Work out the finished part from the listing and answer in its coordinate system (mm). A direction names the side the tool comes from. Coordinates: 2 decimals unless noted, no trailing zeros. Order: outer loops, then holes, each group sorted by start corner. A loop starts at its lowest first (then second) coordinate and runs counter-clockwise, first axis right, second up. Notation, with made-up numbers: M 81,-2 L 119,-2 A17 ccw 119,19 Z; hole C 48,-38.5 d11. An arc over 180 degrees is marked long. Use a Markdown table: item, result.
from build123d import *

# Parameters (mm, degrees)
SKETCH_1_W          = 40.6
SKETCH_1_H          = 20
EXTRUDE_1_DEPTH     = 2
SKETCH_2_W          = 2
SKETCH_2_H          = 20
EXTRUDE_2_DEPTH     = 22
SKETCH_3_R          = 2.5
CUT_EXTRUDE_1_DEPTH = 49.211616857


with BuildPart() as part:
    # 草图1 → 凸台-拉伸1 (new body)
    with BuildSketch(Plane.XY):
        Rectangle(SKETCH_1_W, SKETCH_1_H)
    extrude(amount=EXTRUDE_1_DEPTH)

    # 草图2 → 凸台-拉伸2 (add)
    with BuildSketch(Plane.XY.offset(2)):
        with Locations((-19.3, 0)):
            Rectangle(SKETCH_2_W, SKETCH_2_H)
        with Locations((19.3, 0)):
            Rectangle(SKETCH_2_W, SKETCH_2_H)
    extrude(amount=EXTRUDE_2_DEPTH)

    # 草图3 → 切除-拉伸1 (cut, through all)
    with BuildSketch(Plane.ZY.offset(20.3)):
        with Locations(Location((14, 0, 0), (0, 0, 270))):
            Circle(SKETCH_3_R)
    extrude(amount=-CUT_EXTRUDE_1_DEPTH, mode=Mode.SUBTRACT)


solid = part.part
(1) A cutting plane is placed at A-A (z = 12.5). Determine the outline of the cut face in (x, y), then the cut area to 3 significant figures.
Conclusion:
| item | result |
|---|---|
| outline | M -20.3,-10 L -18.3,-10 L -18.3,-2 L -20.3,-2 Z; M -20.3,2 L -18.3,2 L -18.3,10 L -20.3,10 Z; M 18.3,-10 L 20.3,-10 L 20.3,-2 L 18.3,-2 Z; M 18.3,2 L 20.3,2 L 20.3,10 L 18.3,10 Z |
| area | 64.0 mm2 |
(2) Determine the mould class of faces 1 (the flat face through (18.3, -2.4, 12.8)), 2 (the cylindrical face through (-19.31, 0.54, 11.56)), 3 (the flat face through (0, 0, 2)) for opening direction Z: pulls with the +Z half, pulls with the -Z half, needs draft (parallel to the pull), parting line crosses it, or undercut.
Conclusion:
| item | result |
|---|---|
| face 1 | needs draft |
| face 2 | undercut |
| face 3 | pulls with the +Z half |
(3) Which of the six approach directions +Z, -Z, +X, -X, +Y, -Y give full straight-line access (tool end or side, diameter ignored) to faces 4 (the flat face through (19, 0, 24)), 5 (the flat face through (-18.3, -2.4, 12.8))?
Conclusion:
| item | result |
|---|---|
| face 4 | +Z, +X, -X, +Y, -Y |
| face 5 | +Z, +Y, -Y |
(4) A cutting plane is placed at B-B (y = 0). Determine the outline of the cut face in (x, z), then the cut area to 3 significant figures.
Conclusion:
| item | result |
|---|---|
| outline | M -20.3,0 L 20.3,0 L 20.3,11.5 L 18.3,11.5 L 18.3,2 L -18.3,2 L -18.3,11.5 L -20.3,11.5 Z; M -20.3,16.5 L -18.3,16.5 L -18.3,24 L -20.3,24 Z; M 18.3,16.5 L 20.3,16.5 L 20.3,24 L 18.3,24 Z |
| area | 149 mm2 |
(5) Straight lines are drawn through the part: L1, parallel to Z at x = -19.45, y = 0; L2, parallel to X at y = 6, z = 6.5; L3, parallel to Z at x = -14.5, y = -8.5. For each, find the intervals that lie inside material, in ascending order.
Conclusion:
| item | result |
|---|---|
| L1 | 0 to 11.5, 16.5 to 24 |
| L2 | -20.3 to -18.3, 18.3 to 20.3 |
| L3 | 0 to 2 |
(6) Given P1, Ø1.5, axis at x = 1.5, y = 2.5, coming from the +Z side; P2, Ø8, axis at y = 0, z = 14, coming from the +X side, each flat-ended and moving along its own axis, determine where each tip first touches the part or whether it passes through.
Conclusion:
| item | result |
|---|---|
| P1 | z = 2 |
| P2 | x = 20.3 |
(7) A cutting plane is placed at C-C (z = 18). Determine the outline of the cut face in (x, y), then the cut area to 3 significant figures.
Conclusion:
| item | result |
|---|---|
| outline | M -20.3,-10 L -18.3,-10 L -18.3,10 L -20.3,10 Z; M 18.3,-10 L 20.3,-10 L 20.3,10 L 18.3,10 Z |
| area | 80.0 mm2 |
(8) A cutting plane is placed at D-D (y = 4.5). Determine the outline of the cut face in (x, z), then the cut area to 3 significant figures.
Conclusion:
| item | result |
|---|---|
| outline | M -20.3,0 L 20.3,0 L 20.3,24 L 18.3,24 L 18.3,2 L -18.3,2 L -18.3,24 L -20.3,24 Z |
| area | 169 mm2 |
